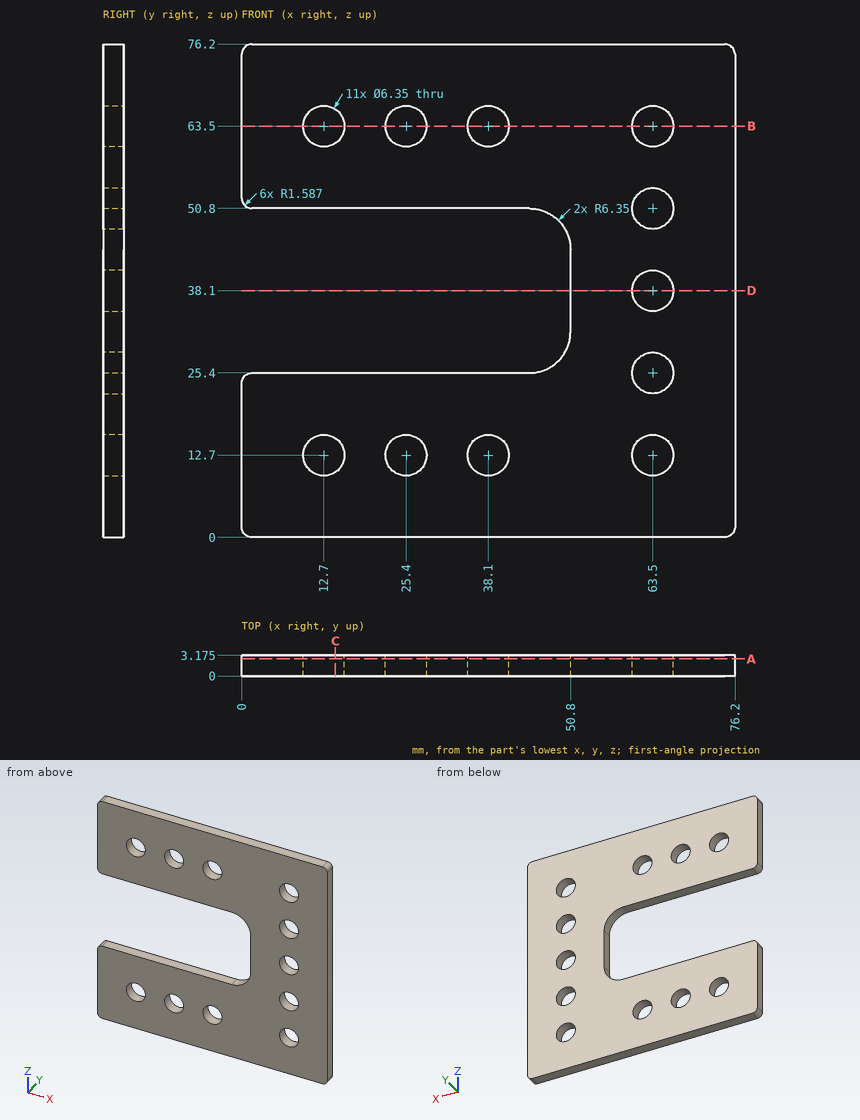
Geometry: see drawing. Coordinates: mm, zero at the bounding-box minimum. Give positions to 0.01 mm unless a question says otherwise; leave off trailing zeros. Loops run counter-clockwise (first coordinate to the right, second up) from the corner with the lowest first, then second, coordinate; pieces in that order, holes last. Notation, with made-up numbers: (-20.75, 46.25) -> (20.25, 46.25) arc R35 ccw to (20.25, 84.25) -> close; hole circle Ø5 at (87, 3.25). An arc over 180 degrees is marked (long way). Answer as a JSON object with one key per item and string values. Group by question number.
Item 1: Cut plane A-A, the plane y = 2.65. State how many separate pieces and enclosed holes the cut face has, and give its area (3 significant figures).
Item 2: Pin query (flat end, axial travel): P1, Ø5.5, axis at x = 25.4, z = 63.5, coming from the +Y side. Return the tip coordinate at first contact, or that it passes through.
Item 3: Cut plane C-C, the plane x = 14.5. Return the cut outline in (y, z) (1 decimal).
Item 4: Cut plane B-B, the plane z = 63.5. Return the cut outline in (x, y) (1 decimal).
Item 5: Line query: probe 1 along X at (y, z) = (1.1, 63.5) (1 decimal); probe 2 along Z at (x, y) = (38, 0.9); probe 3 along Z at (x, y) = (30.5, 1.25). Output: solid intervals per line, ascending.
Item 6: Cut plane D-D, the plane z = 38.1. Return the cut outline in (x, y) (1 decimal).
Checks:
{
 "1": {"separate pieces": "1", "enclosed holes": "11", "area": "4,180 mm²"},
 "2": {"P1": "passes through"},
 "3": {"outline": "(0, 0) -> (3.2, 0) -> (3.2, 10.1) -> (0, 10.1) -> close; (0, 15.3) -> (3.2, 15.3) -> (3.2, 25.4) -> (0, 25.4) -> close; (0, 50.8) -> (3.2, 50.8) -> (3.2, 60.9) -> (0, 60.9) -> close; (0, 66.1) -> (3.2, 66.1) -> (3.2, 76.2) -> (0, 76.2) -> close"},
 "4": {"outline": "(0, 0) -> (9.5, 0) -> (9.5, 3.2) -> (0, 3.2) -> close; (15.9, 0) -> (22.2, 0) -> (22.2, 3.2) -> (15.9, 3.2) -> close; (28.6, 0) -> (34.9, 0) -> (34.9, 3.2) -> (28.6, 3.2) -> close; (41.3, 0) -> (60.3, 0) -> (60.3, 3.2) -> (41.3, 3.2) -> close; (66.7, 0) -> (76.2, 0) -> (76.2, 3.2) -> (66.7, 3.2) -> close"},
 "5": {"probe 1": "x = 0 to 9.5, 15.9 to 22.2, 28.6 to 34.9, 41.3 to 60.3, 66.7 to 76.2", "probe 2": "z = 0 to 9.53, 15.87 to 25.4, 50.8 to 60.33, 66.67 to 76.2", "probe 3": "z = 0 to 25.4, 50.8 to 76.2"},
 "6": {"outline": "(50.8, 0) -> (60.3, 0) -> (60.3, 3.2) -> (50.8, 3.2) -> close; (66.7, 0) -> (76.2, 0) -> (76.2, 3.2) -> (66.7, 3.2) -> close"}
}
